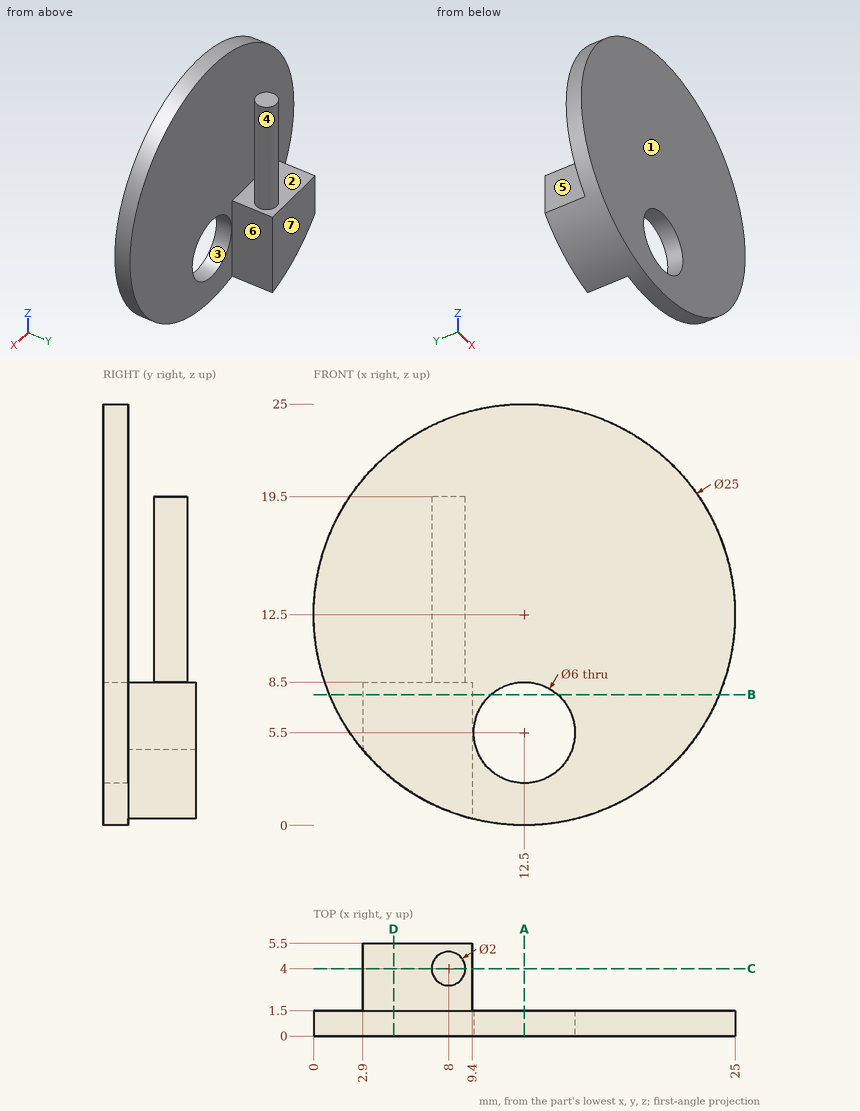
Geometry: see drawing. Coordinates: mm, zero at the bounding-box minimum. A direction names the side the tool comes from. Coordinates: 2 decimals unless noted, no trailing zeros. Loops run counter-clockwise (first coordinate to the right, second up) from the corner with the lowest first, then second, coordinate; pieces in that order, holes last.
Q1. Contact query for flat-ended pins moving along their axis: pin 1 (1 mm diameter, centred on x = 7.5, y = 4.5, fed in from +Z); pin 2 (3 mm diameter, centred on y = 2.5, z = 4, fed in from +X); pin 3 (1 mm diameter, centred on y = 3, z = 3.5, fed in from +X); pin 4 (3.5 mm diameter, centred on x = 12.5, z = 5.5, fed in from -Y). Output: stop coordinate, or through.
Q2. Cut plane A-A (x = 12.5). Output: boundary loops of the cut face in (y, z), then the cut area to 3 significant figures.
Q3. Cut plane C-C (y = 4). Output: boundary loops of the cut face in (x, z), then the cut area to 3 significant figures.
Q4. Cut plane D-D (x = 4.75). Output: boundary loops of the cut face in (y, z), then the cut area to 3 significant figures.
Q5. Material intervals for line 1 (Y direction, x = 9.75, z = 9.5); line 2 (Z direction, x = 5, y = 3.65); line 3 (X direction, y = 4.05, z = 13), sorted ascending.
Q6. Draft query along Y for the marked faces 1, 2, 3 and 4. Return one class per face: +Y half, -Y half, draft (parallel to the pull), parting line (faces both ways), or undercut.
Q7. Cut plane B-B (z = 7.75). Output: boundary loops of the cut face in (x, y), then the cut area to 3 significant figures.
Q8. Set-up query: the marked faces 5, 6 and 7. Return all of +Z, -Z, +X, -X, +Y, -Y with unobstructed straight access to the full face (end or side cutting, diameter ignored); none if empty.
Working result:
1. pin 1: stops at z = 19.5
1. pin 2: stops at x = 22.59
1. pin 3: stops at x = 9.4
1. pin 4: passes through
2. outline: (0, 0) - (1.5, 0) - (1.5, 2.5) - (0, 2.5) - close; (0, 8.5) - (1.5, 8.5) - (1.5, 25) - (0, 25) - close
2. area: 28.5 mm2
3. outline: (2.9, 4.49) arc R12.5 ccw to (9.4, 0.39) - (9.4, 8.5) - (9, 8.5) - (9, 19.5) - (7, 19.5) - (7, 8.5) - (2.9, 8.5) - close
3. area: 64.5 mm2
4. outline: (0, 2.69) - (5.5, 2.69) - (5.5, 8.5) - (1.5, 8.5) - (1.5, 22.31) - (0, 22.31) - close
4. area: 52.7 mm2
5. line 1: y = 0 to 1.5
5. line 2: z = 2.5 to 8.5
5. line 3: x = 7 to 9
6. face 1: -Y half
6. face 2: undercut
6. face 3: draft
6. face 4: undercut
7. outline: (0.94, 0) - (10.52, 0) - (10.52, 1.5) - (9.4, 1.5) - (9.4, 5.5) - (2.9, 5.5) - (2.9, 1.5) - (0.94, 1.5) - close; (14.48, 0) - (24.06, 0) - (24.06, 1.5) - (14.48, 1.5) - close
7. area: 54.7 mm2
8. face 5: +Z, -Z, -X, +Y
8. face 6: +Z, -Z, +X, +Y
8. face 7: +Z, -Z, +X, -X, +Y
